Read the model definition and answer for the solid it produces. Units are mm, in the model's axes. Face numbers are marked on the shaded views. Give positions to 0.01 mm unless a question says otherwise; leave off trailing zeros. Order: outer loops, then holes, each group sorted by start corner. A loop starts at its lowest first (then second) coordinate and runs counter-clockwise, first axis right, second up. Notation, with made-up numbers: M 14,59 L 27,59 A33 cw 27,90 Z; hole C 79.25,49 d7. An arc over 180 degrees is marked long. One line per item, written item: value.
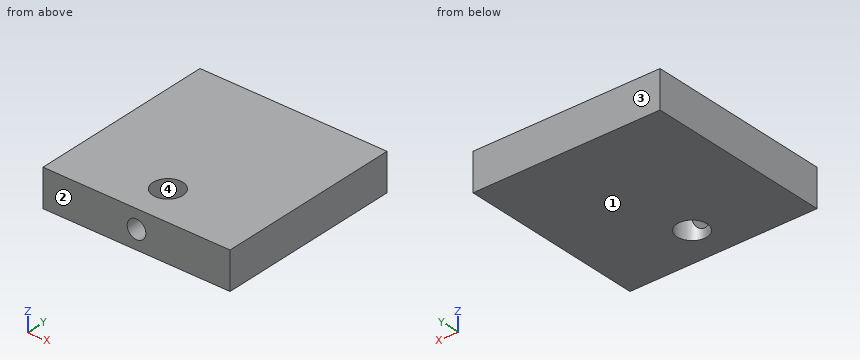
from build123d import *

# Parameters (mm, degrees)
SKETCH_1_W          = 50
SKETCH_1_H          = 50
EXTRUDE_1_DEPTH     = 10
SKETCH_2_R          = 4
CUT_EXTRUDE_1_DEPTH = 10
SKETCH_3_R          = 2.5
CUT_EXTRUDE_2_DEPTH = 10


with BuildPart() as part:
    # Эскиз1 → Бобышка-Вытянуть1 (new body)
    with BuildSketch(Plane.XY):
        with Locations((25, 25)):
            Rectangle(SKETCH_1_W, SKETCH_1_H)
    extrude(amount=EXTRUDE_1_DEPTH)

    # Эскиз2 → Вырез-Вытянуть1 (cut)
    with BuildSketch(Plane.XY.offset(10)):
        with Locations((25, 10)):
            Circle(SKETCH_2_R)
    extrude(amount=-CUT_EXTRUDE_1_DEPTH, mode=Mode.SUBTRACT)

    # Эскиз3 → Вырез-Вытянуть2 (cut)
    with BuildSketch(Plane.XZ):
        with Locations(Location((25, 5, 0), (0, 0, 270))):
            Circle(SKETCH_3_R)
    extrude(amount=-CUT_EXTRUDE_2_DEPTH, mode=Mode.SUBTRACT)


solid = part.part
1) Consider probe 1 along Z at (x, y) = (25, 2); probe 2 along X at (y, z) = (1.75, 5); probe 3 along Y at (x, z) = (25, 3.25). Determine where each line is inside the solid, lowest interval first.
Reported:
probe 1: z = 0 to 2.5, 7.5 to 10
probe 2: x = 0 to 22.5, 27.5 to 50
probe 3: y = 14 to 50
2) Find section B-B, the plane y = 10. Write down the section's boundary in (x, z), plus the area to 3 significant figures.
Reported:
outline: M 0,0 L 21,0 L 21,10 L 0,10 Z; M 29,0 L 50,0 L 50,10 L 29,10 Z
area: 420 mm^2
3) Find section D-D, the plane z = 5. Write down the section's boundary in (x, y).
Reported:
outline: M 0,0 L 22.5,0 L 22.5,6.88 A4 cw long 27.5,6.88 L 27.5,0 L 50,0 L 50,50 L 0,50 Z
4) Determine the mould class of the marked faces 1, 2, 3 and 4 for opening direction Y: +Y half, -Y half, draft (parallel to the pull), parting line (faces both ways), or undercut.
Reported:
face 1: draft
face 2: -Y half
face 3: +Y half
face 4: undercut
5) This flat-tipped pin is pushed along its axis until it touches: pin 1 Ø4 at (y, z) = (13.5, 2) entering from -X. Where does it stop, or does it pass through?
Reported:
pin 1: stops at x = 0
6) Find section A-A, the plane x = 25. Write down the section's boundary in (y, z).
Reported:
outline: M 0,0 L 6,0 L 6,2.5 L 0,2.5 Z; M 0,7.5 L 6,7.5 L 6,10 L 0,10 Z; M 14,0 L 50,0 L 50,10 L 14,10 Z
7) Find section C-C, the plane z = 9. Write down the section's boundary in (x, y).
Reported:
outline: M 0,0 L 50,0 L 50,50 L 0,50 Z; hole C 25,10 d8
